The model under review builds one solid part; all positions refer to its coordinate system, in mm. Face numbers are marked on the shaded views. A direction names the side the tool comes from. Round coordinates to 2 decimals unless told otherwise and drop trailing zeros. Write each loop counter-clockwise with the first axis right and the second up, starting at its lowest first coordinate (ties: lowest second). Pieces come first, ordered by that corner, then holes.
Item 1: Clearance check with flat-ended pins moving along their axes: pin 1 Ø1 at (y, z) = (-68.5, 3.5) entering from -X; pin 2 Ø11 at (x, y) = (40.5, -63) entering from +Z; pin 3 Ø4 at (x, y) = (60.28, -58.23) entering from -Z; pin 4 Ø3 at (x, y) = (63.5, -42.5) entering from +Z. State where each tip first meets the part, or that it passes through.
Item 2: Add section B-B (z = -15.5). Give the boundary of the cut face in (x, y).
Item 3: Draft analysis for pull direction X (two halves, no side actions). For the marked faces 4, 5, 6 and 7, state which applies: +X half, -X half, draft (parallel to the pull), parting line (faces both ways), or undercut.
Item 4: Machinability: for the marked faces 1, 2 and 3, which of the approach directions +Z, -Z, +X, -X, +Y, -Y give a long, thin tool a straight path to every point of the face, cutting with its end or side? Answer none if there is none.
Item 5: Add section A-A (z = 6). Give the boundary of the cut face in (x, y), plus the area to 3 significant figures.
Item 6: To check wall thickness, follow L1, parallel to Z at x = 88, y = -50.5; L2, parallel to Z at x = 107, y = -57; L3, parallel to Z at x = 78, y = -67. State the ranges of each line that lie inside material, in increasing order.
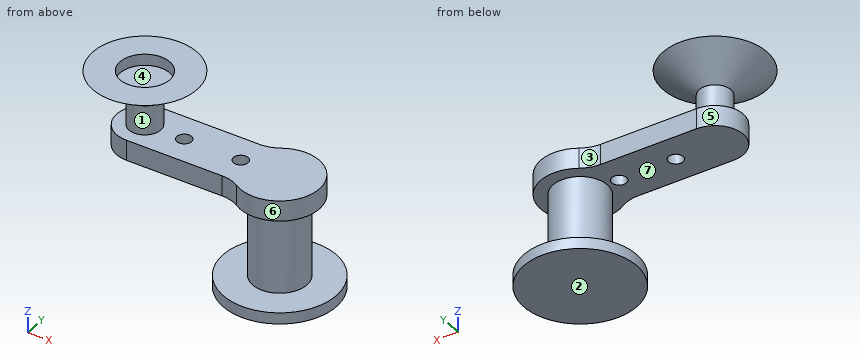
Autodesk Inventor part; units mm, degrees
ref_plane "Plano de trabajo1" through (42.7754, -58.2257, 0) normal (0, -1, 0) x (1, 0, 0)
sketch "Boceto1" plane through (0, 0, 0) normal (0, 0, 1) x (1, 0, 0)
  line L0 (85.4549, -45.7257) -> (42.7754, -45.7257)
  line L1 (42.7754, -70.7257) -> (85.4549, -70.7257)
  arc A0 (42.7754, -45.7257) -> (42.7754, -70.7257) centre (42.7754, -58.2257) ccw
  arc A1 (93.4489, -73.0334) -> (93.4489, -43.418) centre (102.7754, -58.2257) ccw
  arc A2 (85.4549, -45.7257) -> (93.4489, -43.418) centre (85.4549, -30.7257) ccw
  arc A3 (93.4489, -73.0334) -> (85.4549, -70.7257) centre (85.4549, -85.7257) ccw
  circle A4 centre (102.7754, -58.2257) radius 8.1
  circle A5 centre (60.2754, -58.2257) radius 3.25
  circle A6 centre (85.4549, -58.2257) radius 3.25
  line L2 (-16.3205, 1) -> (-59, 1)
  line L3 (-59, -24) -> (-16.3205, -24)
  arc A7 (-59, 1) -> (-59, -24) centre (-59, -11.5) ccw
  line L4 (-59, -21.6036) -> (-67.75, -16.5518)
  line L5 (-67.75, -16.5518) -> (-67.75, -6.4482)
  line L6 (-67.75, -6.4482) -> (-59, -1.3964)
  line L7 (-59, -1.3964) -> (-50.25, -6.4482)
  line L8 (-50.25, -6.4482) -> (-50.25, -16.5518)
  line L9 (-50.25, -16.5518) -> (-59, -21.6036)
  arc A8 (-8.3264, -26.3077) -> (-8.3264, 3.3077) centre (1, -11.5) ccw
  arc A9 (-16.3205, 1) -> (-8.3264, 3.3077) centre (-16.3205, 16) ccw
  arc A10 (-8.3264, -26.3077) -> (-16.3205, -24) centre (-16.3205, -39) ccw
  circle A11 centre (1, -11.5) radius 8.1
  circle A12 centre (-41.5, -11.5) radius 3.25
  circle A13 centre (-16.3205, -11.5) radius 3.25
  line L10 (85.6004, 1.2855) -> (42.9209, 1.2855)
  line L11 (42.9209, -23.7145) -> (85.6004, -23.7145)
  arc A14 (42.9209, 1.2855) -> (42.9209, -23.7145) centre (42.9209, -11.2145) ccw
  line L12 (42.9209, -21.3181) -> (34.1709, -16.2663)
  line L13 (34.1709, -16.2663) -> (34.1709, -6.1627)
  line L14 (34.1709, -6.1627) -> (42.9209, -1.1109)
  line L15 (42.9209, -1.1109) -> (51.6709, -6.1627)
  line L16 (51.6709, -6.1627) -> (51.6709, -16.2663)
  line L17 (51.6709, -16.2663) -> (42.9209, -21.3181)
  arc A15 (93.5944, -26.0222) -> (93.5944, 3.5932) centre (102.9209, -11.2145) ccw
  arc A16 (85.6004, 1.2855) -> (93.5944, 3.5932) centre (85.6004, 16.2855) ccw
  arc A17 (93.5944, -26.0222) -> (85.6004, -23.7145) centre (85.6004, -38.7145) ccw
  circle A18 centre (102.9209, -11.2145) radius 8.1
  circle A19 centre (60.4209, -11.2145) radius 3.25
  circle A20 centre (85.6004, -11.2145) radius 3.25
  circle A21 centre (42.7754, -58.2257) radius 7
  line L18 (-15.6185, -45.6026) -> (-58.298, -45.6026)
  line L19 (-58.298, -70.6026) -> (-15.6185, -70.6026)
  arc A22 (-58.298, -45.6026) -> (-58.298, -70.6026) centre (-58.298, -58.1026) ccw
  arc A23 (-7.6244, -72.9103) -> (-7.6244, -43.2949) centre (1.702, -58.1026) ccw
  arc A24 (-15.6185, -45.6026) -> (-7.6244, -43.2949) centre (-15.6185, -30.6026) ccw
  arc A25 (-7.6244, -72.9103) -> (-15.6185, -70.6026) centre (-15.6185, -85.6026) ccw
  circle A26 centre (1.702, -58.1026) radius 8.1
  circle A27 centre (-40.798, -58.1026) radius 3.25
  circle A28 centre (-15.6185, -58.1026) radius 3.25
  circle A29 centre (-58.298, -58.1026) radius 7
  point P0 (90.5279, -45.7257)
  point P1 (90.5279, -70.7257)
  point P2 (-11.2474, 1)
  point P3 (-11.2474, -24)
  point P4 (90.6734, 1.2855)
  point P5 (90.6734, -23.7145)
  point P6 (-10.5454, -45.6026)
  point P7 (-10.5454, -70.6026)
extrude "Extrusión1" add sketch "Boceto1" along normal blind 9 contours A2 A1 A3 L1 A0 L0
sketch "Boceto2" plane through (0, 0, 0) normal (0, 0, -1) x (-1, 0, 0)
  circle A0 centre (-102.7754, -58.2257) radius 8.1
  circle A1 centre (-102.7754, -58.2257) radius 12
  point P0 (0, 0)
  dimension "d13" = 24
extrude "Extrusión2" add sketch "Boceto2" along normal blind 36 and the other way blind 9 contours A0 | A1
sketch "Boceto3" plane through (102.7754, -58.2257, -36) normal (0, 0, -1) x (-1, 0, 0)
  circle A0 centre (0, 0) radius 25
  point P0 (102.7754, 58.2257)
  dimension "d16" = 50
extrude "Extrusión3" add sketch "Boceto3" along normal blind 5
ref_plane "Plano de trabajo1" through (42.7754, -58.2257, 0) normal (0, -1, 0) x (1, 0, 0)
sketch "Boceto7" plane through (42.7754, -58.2257, 0) normal (0, -1, 0) x (1, 0, 0)
  line L0 (-7, 0) -> (7, 0)
  line L1 (7, 9) -> (7, 0)
  line L2 (-7, 0) -> (7, 0)
  line L3 (7, 0) -> (7, 9)
  line L4 (-7, 9) -> (-7, 0)
  line L5 (-7, 9) -> (-7, 22)
  line L6 (7, 22) -> (7, 9)
  line L7 (23, 33) -> (-23, 33)
  line L8 (7, 22) -> (23, 33)
  line L9 (-7, 22) -> (-23, 33)
  line L10 (0, -1.9215) -> (0, 41.7304)
  point P0 (-42.7754, 0)
  point P1 (0, 9)
  point P2 (0, 0)
  point P3 (0, 33)
  dimension "d23" = 14
  dimension "d24" = 13
  dimension "d38" = 46
  dimension "d39" = 11
revolve "Revolución1" add sketch "Boceto7" angle 360 about axis through (42.7754, -58.2257, -1.9215) along (0, 0, 1) contours L4 L5 L9 L7 L10 L0
sketch "Boceto8" plane through (42.7754, -58.2257, 33) normal (0, 0, 1) x (1, 0, 0)
  circle A0 centre (0, 0) radius 11
  point P0 (-42.7754, 58.2257)
  dimension "d29" = 22
extrude "Extrusión5" cut sketch "Boceto8" against normal blind 5
properties part number "Herramienta1"
Numbers:
1. pin 1: stops at x = 34.98
1. pin 2: stops at z = 28
1. pin 3: stops at z = 27.85
1. pin 4: passes through
2. outline: circle Ø24 at (102.78, -58.23)
3. face 4: undercut
3. face 5: -X half
3. face 6: parting line
3. face 7: draft
4. face 1: none
4. face 2: -Z, +X, -X, +Y, -Y
4. face 3: +Z, -X, +Y
5. outline: (42.78, -70.73) - (85.45, -70.73) arc R15 cw to (93.45, -73.03) arc R17.5 ccw (long way) to (93.45, -43.42) arc R15 cw to (85.45, -45.73) - (42.78, -45.73) arc R12.5 ccw to start; hole circle Ø6.5 at (60.28, -58.23); hole circle Ø6.5 at (85.45, -58.23)
5. area: 2,250 mm2
6. L1: z = -41 to -36, 0 to 9
6. L2: z = -41 to 9
6. L3: z = 0 to 9
